Can you work these out from the model? Positions are in its coordinate system, mm. A direction names the side the tool comes from. Give positions to 0.01 mm unless a question says otherwise; leave off trailing zeros. Write each loop counter-clockwise with the first axis right and the second up, starting at its lowest first coordinate (ties: lowest second). Pieces come first, ordered by that corner, then holes.
```python
from build123d import *

# Parameters (mm, degrees)
BASEHEAD_DEPTH = 15
SKETCH4_W      = 0.8
SKETCH4_H      = 13.171361037


# Read off the part's stored shape, not the designer's step: HeadChamfer
with BuildPart() as part:
    # Sketch1 → BaseHead (new body)
    with BuildSketch(Plane(origin=(0, 0, 0), x_dir=(0, 0, -1), z_dir=(1, 0, 0))):
        Polygon((20.5, 11.835680518), (20.5, -11.835680518), (0, -23.671361037), (-20.5, -11.835680518), (-20.5, 11.835680518), (0, 23.671361037), align=None)
    extrude(amount=BASEHEAD_DEPTH)

    # HeadChamfer outline → HeadChamfer (revolve, cut)
    with BuildSketch(Plane.YX):
        Polygon((23.671361268, 1.830986282), (20.499999702, -1.72e-07), (23.671361268, -1.72e-07), align=None)
    revolve(axis=Axis((0, 0, 0), (1, 0, 0)), mode=Mode.SUBTRACT)

    # HeadChamfer 2 outline → HeadChamfer 2 (revolve)
    with BuildSketch(Plane.YX):
        Polygon((12, 15), (12, 103.352), (10.352, 105), (0, 105), (0, 15), align=None)
    revolve(axis=Axis((0, 0, 0), (1, 0, 0)))

    # Sketch4 → BearingFace (revolve, cut)
    with BuildSketch(Plane.XY, mode=Mode.PRIVATE) as bearingface_sk:
        with Locations((14.6, 27.085680519)):
            Rectangle(SKETCH4_W, SKETCH4_H)
    revolve(bearingface_sk.sketch.rotate(Axis((0, 0, 0), (1, 0, 0)), 90), axis=Axis((0, 0, 0), (1, 0, 0)), mode=Mode.SUBTRACT)


solid = part.part
```
1) Please list where these lines run through material, in increasing order: L1, parallel to X at y = -7, z = -11.5; L2, parallel to Y at x = 34, z = 8; L3, parallel to Y at x = 90, z = 9.
Values follow:
L1: x = 0 to 15
L2: y = -8.94 to 8.94
L3: y = -7.94 to 7.94
2) For faces 1 (the face through (14.2, -10.2, 18.4)), 2 (the face through (59.79, -11.99, 0.53)), 3 (the face through (14.2, 11, -18)), 4 (the face through (14.2, 11, 18)), 5 (the face through (14.2, 21, 0)), which set-ups out of +Z, -Z, +X, -X, +Y, -Y let a thin tool reach every point of the face, with its end or its side?
Values follow:
face 1: +Z, +X, -Y
face 2: +X
face 3: -Z, +X, +Y
face 4: +Z, +X, +Y
face 5: +X, +Y
3) If we mould it in two halves opening along Y, with no side actions, what happens to faces 6 (the face through (7.001, -17.836, 10.106)), 7 (the face through (14.61, 12.47, -16.27)), 8 (the face through (15, -9, 9))? For each: +Y half, -Y half, draft (parallel to the pull), parting line (faces both ways), or undercut.
Values follow:
face 6: -Y half
face 7: parting line
face 8: draft
4) For pin 1 Ø8 at (x, y) = (48, -4.5) entering from -Z; pin 2 Ø4 at (x, z) = (45, -9) entering from +Y; pin 3 Ø3 at (x, z) = (86.5, -8) entering from -Y, each with a flat end and sliding along its axis, tell me the tip position at first contact or that it passes through.
Values follow:
pin 1: stops at z = -11.99
pin 2: stops at y = 9.75
pin 3: stops at y = -10.09
5) Suppose I cut it at A-A on x = 82.5. Write out the boundary of the cut face in (y, z), plus the area to 3 significant figures.
Values follow:
outline: circle Ø24 at (0, 0)
area: 452 mm2
